```python
from build123d import *

# Parameters (mm, degrees)
F0_W     = 20
F0_H     = 20
F1_DEPTH = 3
F3_DEPTH = 5
F5_COUNT = 4
F6_R     = 1.5


with BuildPart() as f1:
    # F0 (on Top) → F1 (new body)
    with BuildSketch(Plane.XY):
        Rectangle(F0_W, F0_H)
    extrude(amount=F1_DEPTH)

    # F2 (on face) → F3 (join)
    with BuildSketch(Plane(origin=(0, 0, 0), x_dir=(1, 0, 0), z_dir=(0, 0, -1))):
        with BuildLine():
            Line((-2.5, -8), (-2.5, -10))
            Line((-2.5, -10), (2.5, -10))
            Line((2.5, -10), (2.5, -8))
            Line((2.5, -8), (4.5, -8))
            ThreePointArc((4.5, -8), (4.8535533906, -7.8535533906), (5, -7.5))
            Line((5, -7.5), (5, -7))
            ThreePointArc((5, -7), (4.8535533906, -6.6464466094), (4.5, -6.5))
            Line((4.5, -6.5), (-4.5, -6.5))
            ThreePointArc((-4.5, -6.5), (-4.8535533906, -6.6464466094), (-5, -7))
            Line((-5, -7), (-5, -7.5))
            ThreePointArc((-5, -7.5), (-4.8535533906, -7.8535533906), (-4.5, -8))
            Line((-4.5, -8), (-2.5, -8))
        make_face()
    extrude(amount=F3_DEPTH)

    # F5: F1 ×4 about axis
    f5_axis = Axis((0, 0, -8.8594034314), (0, 0, -1))


with BuildPart() as f1_1:
    add(f1.part)
    for i in range(1, F5_COUNT):
        add(f1.part.rotate(f5_axis, i * 360 / F5_COUNT))

    # F6
    f6_edges = [f1_1.edges().sort_by_distance(p)[0] for p in [
        (-10, 0, 3),
        (0, 10, 3),
        (0, -10, 3),
        (10, 0, 3),
        (10, -10, 1.5),
        (10, 10, 1.5),
        (-10, 10, 1.5),
        (-10, -10, 1.5),
    ]]
    fillet(f6_edges, radius=F6_R)


solid = f1_1.part
```
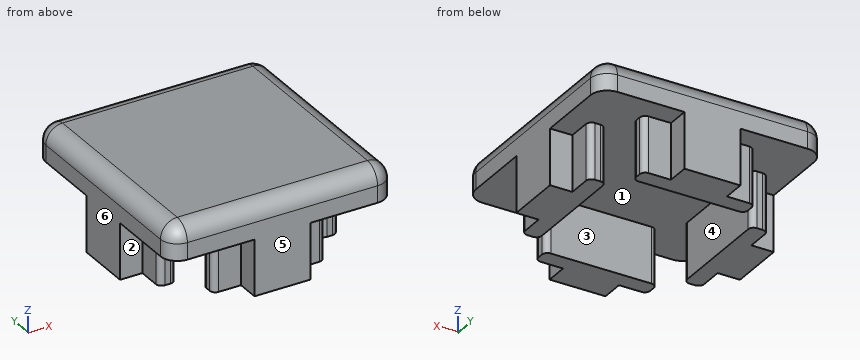
Verification items for the finished model (mm, model axes). Face numbers are marked on the shaded views. A direction names the side the tool comes from. Coordinates: 2 decimals unless noted, no trailing zeros. Loops run counter-clockwise (first coordinate to the right, second up) from the corner with the lowest first, then second, coordinate; pieces in that order, holes last. Notation, with made-up numbers: (81, 43) - (125, 43) arc R23 cw to (125, 82) - close; hole circle Ø1 at (-3, 16.5). An arc over 180 degrees is marked (long way). Put each result on its own line as item: value.
Item 1: Draft check along X on the marked faces 4, 5 and 6. Enter one of: pulls with the +X half, pulls with the -X half, needs draft (parallel to the pull), parting line crosses it, or undercut.
Conclusion:
face 4: undercut
face 5: needs draft
face 6: pulls with the -X half
Item 2: Section check B-B (y = -2.25). Enter the section's corners in (x, z).
Conclusion:
outline: (-10, -5) - (-6.5, -5) - (-6.5, 0) - (6.5, 0) - (6.5, -5) - (10, -5) - (10, 1.5) arc R1.5 ccw to (8.5, 3) - (-8.5, 3) arc R1.5 ccw to (-10, 1.5) - close
Item 3: Section check A-A (x = -2.75). Enter the section's corners in (y, z).
Conclusion:
outline: (-10, 0) - (-8, 0) - (-8, -5) - (-6.5, -5) - (-6.5, 0) - (6.5, 0) - (6.5, -5) - (8, -5) - (8, 0) - (10, 0) - (10, 1.5) arc R1.5 ccw to (8.5, 3) - (-8.5, 3) arc R1.5 ccw to (-10, 1.5) - close
Item 4: Scan lines: line 1 along X through (y, z) = (4.25, -2.25); line 2 along Y through (x, z) = (-1.5, -1.75). Record each from-to range of solid material in increasing order.
Conclusion:
line 1: x = -8 to -6.5, 6.5 to 8
line 2: y = -10 to -6.5, 6.5 to 10
Item 5: Gauge pin test, flat ends, axial feed: pin 1 Ø1.6 at (y, z) = (-9, -2) entering from -X; pin 2 Ø1 at (x, z) = (-3.5, -3) entering from +Y; pin 3 Ø1.6 at (y, z) = (-3, -2.5) entering from +X; pin 4 Ø1.6 at (x, z) = (-9, -3.5) entering from +Y. Record the tip position at first contact, or that the pin passes through.
Conclusion:
pin 1: stops at x = -2.5
pin 2: stops at y = 8
pin 3: stops at x = 10
pin 4: stops at y = 2.5
Item 6: Set-up check for the marked faces 1, 2 and 3: record each of +Z, -Z, +X, -X, +Y, -Y from which the full face is reachable in a straight line by a thin tool's end or side.
Conclusion:
face 1: -Z
face 2: -Z, -X, -Y
face 3: -Z, +X, -X
Item 7: Section check C-C (z = -1). Give the number of separate pieces and of enclosed holes in the cut face, then the cut area to 3 significant figures.
Conclusion:
separate pieces: 4
enclosed holes: 0
area: 99.1 mm2
